Autodesk Inventor part; units mm, degrees
ref_plane "YZ Plane" through (0, 0, 0) normal (1, 0, 0) x (0, 1, 0)
ref_plane "XZ Plane" through (0, 0, 0) normal (0, 1, 0) x (-1, 0, 0)
ref_plane "XY Plane" through (0, 0, 0) normal (0, 0, 1) x (1, 0, 0)
sketch "Sketch1" plane through (0, 0, 0) normal (1, 0, 0) x (0, 1, 0)
  line L0 (6.35, 64.4848) -> (0, 64.4848)
  line L1 (0, 64.4848) -> (0, -37.1152)
  line L2 (0, -37.1152) -> (6.35, -37.1152)
  line L3 (38.1, -11.7152) -> (38.1, 39.0848)
  line L4 (38.1, 39.0848) -> (6.35, 39.0848)
  line L5 (38.1, -11.7152) -> (6.35, -11.7152)
  line L6 (6.35, -37.1152) -> (6.35, -11.7152)
  line L7 (6.35, 39.0848) -> (6.35, 64.4848)
  point P0 (0, 0)
  dimension "d1" = 101.6
  dimension "d3" = 25.4
  dimension "d4" = 25.4
extrude "Extrusion1" add sketch "Sketch1" along normal blind 12.7
sketch "Sketch2" plane through (0, 6.35, 64.4848) normal (0, 1, 0) x (1, 0, 0)
  line L0 (0, 0) -> (12.7, 0)
  line L1 (12.7, 25.4) -> (12.7, 0)
  line L2 (0, 101.6) -> (12.7, 101.6)
  line L3 (0, 101.6) -> (0, 76.2)
  point P0 (0, 64.4848)
  point P1 (6.35, 12.7)
  point P2 (6.35, 88.9)
  dimension "d7" = 12.7
  dimension "d8" = 6.35
  dimension "d9" = 12.7
  dimension "d10" = 6.35
hole "Hole1" at (6.35, 6.35, 51.7848) at (6.35, 6.35, -24.4152) direction (0, -1, 0) diameter 4.4958 end through all
sketch "Sketch3" plane through (0, 38.1, 39.0848) normal (0, 1, 0) x (1, 0, 0)
  line L0 (-8.738, -5.974) -> (3.683, -5.974)
  line L1 (3.683, -5.974) -> (3.683, 55.8495)
  line L2 (3.683, 55.8495) -> (-8.738, 55.8495)
  line L3 (-8.738, 55.8495) -> (-8.738, -5.974)
  line L4 (0, 50.8) -> (0, 0)
  point P0 (0, 39.0848)
  dimension "d18" = 3.683
extrude "Extrusion2" cut sketch "Sketch3" against normal blind 31.75
sketch "Sketch4" plane through (12.7, 0, 0) normal (1, 0, 0) x (0, 0, -1)
  circle A0 centre (-13.6848, 22.225) radius 3.81
  line L0 (11.7152, 38.1) -> (-39.0848, 38.1)
  line L1 (11.7152, 6.35) -> (11.7152, 38.1)
  point P0 (0, 0)
  dimension "d21" = 15.875
  dimension "d22" = 25.4
  dimension "d25" = 7.62
extrude "Extrusion3" cut sketch "Sketch4" against normal blind 25.4
sketch "Sketch5" plane through (12.7, 0, 0) normal (1, 0, 0) x (0, 0, -1)
  circle A0 centre (-13.6848, 22.225) radius 3.81
  point P0 (0, 0)
  point P1 (-21.6858, 30.226)
  point P2 (-5.6838, 30.226)
  point P3 (-5.6838, 14.224)
  point P4 (-21.6858, 14.224)
  dimension "d26" = 8.001
  dimension "d27" = 8.001
  dimension "d28" = 0
  dimension "d29" = 0
  dimension "d30" = 8.001
  dimension "d31" = 8.001
  dimension "d32" = 0
  dimension "d33" = 0
hole "Hole2" at (12.7, 30.226, 21.6858) at (12.7, 30.226, 5.6838) at (12.7, 14.224, 5.6838) at (12.7, 14.224, 21.6858) direction (-1, 0, 0) diameter 2.4384 end through all
fillet "Fillet1" radius 12.7 2 edges at (8.1915, 38.1, 39.0848) (8.1915, 38.1, -11.7152)
properties part number "SliderMotorMount"
Source: CAD feature listing. Evaluate the final solid. Frame: model axes, mm. A direction names the side the tool comes from. Round coordinates to 2 decimals unless told otherwise and drop trailing zeros. Loops run counter-clockwise (first coordinate to the right, second up) from the corner with the lowest first, then second, coordinate; pieces in that order, holes last. Notation, with made-up numbers: M -4.5,-28 L 34.5,-28 A27 ccw 34.5,8 Z; hole C 73.5,-32 d10. An arc over 180 degrees is marked long. Put each result on its own line as item: value.
(1) Section B-B, the plane y = 7.5. Return loops of the section in (x, z).
Solutions:
outline: M 3.68,-11.72 L 12.7,-11.72 L 12.7,39.08 L 3.68,39.08 Z
(2) First-contact query: pin 1 (4 mm diameter, centred on x = 9, z = -19, fed in from +Y); pin 2 (10 mm diameter, centred on y = 20.5, z = 36.5, fed in from -X); pin 3 (7 mm diameter, centred on y = 22.22, z = 13.68, fed in from +X); pin 4 (4.5 mm diameter, centred on x = 8.5, y = 19, fed in from -Z). Flat tips, straight axial feed; report the tip coordinate or a pass-through.
Solutions:
pin 1: y = 6.35
pin 2: x = 3.68
pin 3: through
pin 4: z = -11.72
(3) Pull-direction query (Y, two-part tool) for faces 1 (the face through (8.13, 13.86, 4.52)), 2 (the face through (6, 0, 14)), 3 (the face through (8.255, 34.281, -8.094)); classes: released by +Y, released by -Y, zero draft, split by the parting line, or undercut.
Solutions:
face 1: undercut
face 2: released by -Y
face 3: released by +Y
(4) Section C-C, the plane z = 0. Return loops of the section in (x, y), and give its area (3 significant figures).
Solutions:
outline: M 0,0 L 12.7,0 L 12.7,38.06 L 3.68,38.06 L 3.68,6.35 L 0,6.35 Z
area: 367 mm²
(5) Section D-D, the plane z = 48.5. Return loops of the section in (x, y).
Solutions:
outline: M 0,0 L 12.7,0 L 12.7,6.35 L 0,6.35 Z
(6) Access query for faces 4 (the face through (8, 16, -11.715)), 5 (the face through (3, 6.35, 13)), 6 (the face through (8, 16, 39.085)). Directions: +Z, -Z, +X, -X, +Y, -Y. A direction counts if a zero-diameter tool reaches every point of the face in a straight line with its end or side. Return the directions, or none.
Solutions:
face 4: -Z, +X, -X, +Y
face 5: -X, +Y
face 6: +Z, +X, -X, +Y
(7) Ray query, line 1 (Y direction, x = 7.25, z = 21); line 2 (Y direction, x = 8, z = 42); line 3 (Y direction, x = 10.5, z = 15). Return the intervals inside material, ascending. Write a range as [from, to].
Solutions:
line 1: [0, 13.22], [15.23, 29.22], [31.23, 38.1]
line 2: [0, 6.35]
line 3: [0, 18.65], [25.8, 38.1]
(8) Section A-A, the plane x = 6.35. Return loops of the section in (y, z) (3 decimals).
Solutions:
outline: M 0,-37.115 L 6.35,-37.115 L 6.35,-26.663 L 0,-26.663 Z; M 0,-22.167 L 6.35,-22.167 L 6.35,-11.715 L 25.4,-11.715 A12.7 ccw 38.1,0.985 L 38.1,26.385 A12.7 ccw 25.4,39.085 L 6.35,39.085 L 6.35,49.537 L 0,49.537 Z; M 0,54.033 L 6.35,54.033 L 6.35,64.485 L 0,64.485 Z; hole C 14.224,5.684 d2.438; hole C 14.224,21.686 d2.438; hole C 22.225,13.685 d7.62; hole C 30.226,5.684 d2.438; hole C 30.226,21.686 d2.438
